Input: part model. Units: mm. Frame: model coordinates. Coordinates: 2 decimals unless noted, no trailing zeros. Write each loop counter-clockwise with the first axis right and the second up, starting at its lowest first coordinate (ties: lowest second). Pieces come first, ordered by that corner, then holes. Notation, with made-up numbers: M -26.5,-20.5 L 4.5,-20.5 A23 cw 4.5,13.5 Z; hole C 53.5,16 d5. An arc over 180 degrees is marked long. Answer as a JSON object with one key per item and string values. Group by question number.
from build123d import *

# Parameters (mm, degrees)
F1_DEPTH  = 6.35
F2_W      = 25.4
F2_H      = 10.16
F3_DEPTH  = 1.27
F4_R      = 2.54
F5_DEPTH  = 25.4
F6_R      = 2.54
F7_DEPTH  = 25.4
F8_R      = 1.905
F9_DEPTH  = 254
F10_R     = 3.17499
F11_R     = 1.26999
F12_W     = 10.7186027977
F12_H     = 11.3617175813
F13_DEPTH = 2.54
F14_W     = 7.8115976844
F14_H     = 7.0746540246
F15_DEPTH = 2.54


# Not quite as in the source:
# - a fillet or chamfer is up to 0.001 mm smaller than in the source, because OpenCascade refuses the exact size


with BuildPart() as f1:
    # F0 (on Top) → F1 (new body)
    with BuildSketch(Plane.XY):
        Polygon((-53.3815915518, -2.0840423941), (-101.6415915518, -2.0840423941), (-101.6415915518, -51.6140423941), (-101.6415915518, -59.2340423941), (-53.3815915518, -59.2340423941), (-53.3815915518, -51.6140423941), (86.3184084482, -51.6140423941), (86.3184084482, -59.2340423941), (134.5784084482, -59.2340423941), (134.5784084482, -51.6140423941), (134.5784084482, -2.0840423941), (86.3184084482, -2.0840423941), align=None)
    extrude(amount=F1_DEPTH)

    # F2 (on face) → F3 (cut)
    with BuildSketch(Plane.XY.offset(6.35)):
        with Locations((-88.9415915518, -7.1640423941)):
            Rectangle(F2_W, F2_H)
        with Locations((121.8784084482, -7.1640423941)):
            Rectangle(F2_W, F2_H)
    extrude(amount=-F3_DEPTH, mode=Mode.SUBTRACT)

    # F4 (on face) → F5 (cut)
    with BuildSketch(Plane.XY.offset(5.08)):
        with Locations((-97.8315915518, -7.1640423941)):
            Circle(F4_R)
        with Locations((-81.0675915518, -7.1640423941)):
            Circle(F4_R)
    extrude(amount=-F5_DEPTH, mode=Mode.SUBTRACT)

    # F6 (on face) → F7 (cut)
    with BuildSketch(Plane.XY.offset(5.08)):
        with Locations((130.7684084482, -7.1640423941)):
            Circle(F6_R)
        with Locations((114.0044084482, -7.1640423941)):
            Circle(F6_R)
    extrude(amount=-F7_DEPTH, mode=Mode.SUBTRACT)

    # F8 (on face) → F9 (cut, symmetric)
    with BuildSketch(Plane.YZ.offset(-53.3815915518)):
        with Locations((-55.4240423941, 3.175)):
            Circle(F8_R)
    extrude(amount=F9_DEPTH, both=True, mode=Mode.SUBTRACT)

    # F10 (radius 3.175 in the source; OpenCascade refuses exactly that, so slightly less here)
    f10_edges = [f1.edges().sort_by_distance(p)[0] for p in [
        (-77.511592, -59.234042, 6.35),
        (-77.511592, -59.234042, 0),
        (110.448408, -59.234042, 6.35),
        (110.448408, -59.234042, 0),
    ]]
    fillet(f10_edges, radius=F10_R)

    # F11 (radius 1.27 in the source; OpenCascade refuses exactly that, so slightly less here)
    f11_edges = [f1.edges().sort_by_distance(p)[0] for p in [
        (-101.641592, -34.151547, 6.35),
        (134.578408, -34.151547, 6.35),
    ]]
    fillet(f11_edges, radius=F11_R)

    # F12 (on face) → F13 (cut)
    with BuildSketch(Plane(origin=(-101.6415915518, 0, 0), x_dir=(0, -1, 0), z_dir=(-1, 0, 0))):
        with Locations((56.973343793, 2.878480358)):
            Rectangle(F12_W, F12_H)
    extrude(amount=-F13_DEPTH, mode=Mode.SUBTRACT)

    # F14 (on face) → F15 (cut)
    with BuildSketch(Plane.YZ.offset(134.5784084482)):
        with Locations((-55.5198412363, 2.9937927611)):
            Rectangle(F14_W, F14_H)
    extrude(amount=-F15_DEPTH, mode=Mode.SUBTRACT)


solid = f1.part
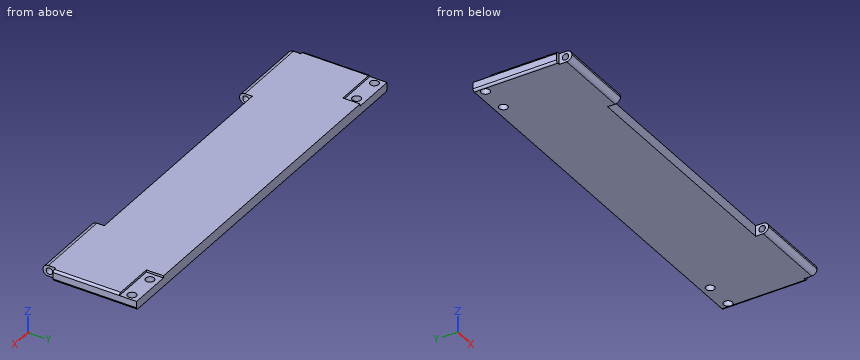
Q1. Pin query (flat end, axial travel): pin 1 Ø1.5 at (x, z) = (70.5, 2) entering from -Y; pin 2 Ø8 at (x, y) = (114, -7.16) entering from +Z; pin 3 Ø3.5 at (y, z) = (-55.42, 3.18) entering from +X; pin 4 Ø1 at (x, z) = (-67, 1) entering from -Y. Return the tip coordinate at first contact, or that it passes through.
Q2. Section B-B, the plane x = -17.5. Return the cut outline in (y, z).
Q3. Line query: line 1 (X direction, y = -53.5, z = 1); line 2 (X direction, y = -9, z = 2.75); line 3 (Y direction, x = 26, z = 3.5). Output: solid intervals per line, ascending. Write a range as from..to.
Filled in:
{
 "1": {"pin 1": "y = -51.61", "pin 2": "z = 5.08", "pin 3": "through", "pin 4": "y = -58.76"},
 "2": {"outline": "M -51.61,0 L -2.08,0 L -2.08,6.35 L -51.61,6.35 Z"},
 "3": {"line 1": "-99.1..-53.38, 86.32..132.04", "line 2": "-101.64..-99.59, -96.08..-82.82, -79.31..112.25, 115.76..129.01, 132.52..134.58", "line 3": "-51.61..-2.08"}
}
